Autodesk Inventor part; units mm, degrees
ref_plane "YZ Plane" through (0, 0, 0) normal (1, 0, 0) x (0, 1, 0)
ref_plane "XZ Plane" through (0, 0, 0) normal (0, 1, 0) x (-1, 0, 0)
ref_plane "XY Plane" through (0, 0, 0) normal (0, 0, 1) x (1, 0, 0)
sketch "スケッチ1" plane through (0, 0, 0) normal (0, 0, 1) x (1, 0, 0)
  arc A0 (-3.8168, 9.7817) -> (-3.6234, 7.4117) centre (4.2362, 9.2462) ccw
  arc A1 (-3.6234, 7.4117) -> (-4.2231, 7.0872) centre (0, 0) ccw
  arc A2 (-4.2231, 7.0872) -> (-6.1013, 8.5454) centre (-10.0576, 1.5108) ccw
  arc A3 (-6.1013, 8.5454) -> (-6.7861, 8.0124) centre (0, 0) ccw
  arc A4 (-6.7861, 8.0124) -> (-5.8336, 5.8336) centre (1.0044, 10.1207) ccw
  arc A5 (-5.8336, 5.8336) -> (-6.2954, 5.332) centre (0, 0) ccw
  arc A6 (-6.2954, 5.332) -> (-8.5454, 6.1013) centre (-10.0032, -1.8368) ccw
  arc A7 (-8.5454, 6.1013) -> (-9.0201, 5.3748) centre (0, 0) ccw
  arc A8 (-9.0201, 5.3748) -> (-7.4117, 3.6234) centre (-2.3362, 9.8985) ccw
  arc A9 (-7.4117, 3.6234) -> (-7.6856, 2.9989) centre (0, 0) ccw
  arc A10 (-7.6856, 2.9989) -> (-10.0635, 2.996) centre (-8.8648, -4.9853) ccw
  arc A11 (-10.0635, 2.996) -> (-10.2765, 2.1548) centre (0, 0) ccw
  arc A12 (-10.2765, 2.1548) -> (-8.1866, 1.0205) centre (-5.4236, 8.6036) ccw
  arc A13 (-8.1866, 1.0205) -> (-8.243, 0.3409) centre (0, 0) ccw
  arc A14 (-8.243, 0.3409) -> (-10.491, -0.4339) centre (-6.7658, -7.5935) ccw
  arc A15 (-10.491, -0.4339) -> (-10.4194, -1.2988) centre (0, 0) ccw
  arc A16 (-10.4194, -1.2988) -> (-8.0744, -1.693) centre (-7.9233, 6.3764) ccw
  arc A17 (-8.0744, -1.693) -> (-7.907, -2.354) centre (0, 0) ccw
  arc A18 (-7.907, -2.354) -> (-9.7817, -3.8168) centre (-3.9336, -9.3789) ccw
  arc A19 (-9.7817, -3.8168) -> (-9.4331, -4.6116) centre (0, 0) ccw
  arc A20 (-9.4331, -4.6116) -> (-7.0872, -4.2231) centre (-9.5644, 3.4582) ccw
  arc A21 (-7.0872, -4.2231) -> (-6.7143, -4.7939) centre (0, 0) ccw
  arc A22 (-6.7143, -4.7939) -> (-8.0124, -6.7861) centre (-0.6751, -10.148) ccw
  arc A23 (-8.0124, -6.7861) -> (-7.4246, -7.4246) centre (0, 0) ccw
  arc A24 (-7.4246, -7.4246) -> (-5.332, -6.2954) centre (-10.1691, 0.1652) ccw
  arc A25 (-5.332, -6.2954) -> (-4.7939, -6.7143) centre (0, 0) ccw
  arc A26 (-4.7939, -6.7143) -> (-5.3748, -9.0201) centre (2.6565, -9.8173) ccw
  arc A27 (-5.3748, -9.0201) -> (-4.6116, -9.4331) centre (0, 0) ccw
  arc A28 (-4.6116, -9.4331) -> (-2.9989, -7.6856) centre (-9.6717, -3.1456) ccw
  arc A29 (-2.9989, -7.6856) -> (-2.354, -7.907) centre (0, 0) ccw
  arc A30 (-2.354, -7.907) -> (-2.1548, -10.2765) centre (5.7003, -8.4228) ccw
  arc A31 (-2.1548, -10.2765) -> (-1.2988, -10.4194) centre (0, 0) ccw
  arc A32 (-1.2988, -10.4194) -> (-0.3409, -8.243) centre (-8.1263, -6.1156) ccw
  arc A33 (-0.3409, -8.243) -> (0.3409, -8.243) centre (0, 0) ccw
  arc A34 (0.3409, -8.243) -> (1.2988, -10.4194) centre (8.1263, -6.1156) ccw
  arc A35 (1.2988, -10.4194) -> (2.1548, -10.2765) centre (0, 0) ccw
  arc A36 (2.1548, -10.2765) -> (2.354, -7.907) centre (-5.7003, -8.4228) ccw
  arc A37 (2.354, -7.907) -> (2.9989, -7.6856) centre (0, 0) ccw
  arc A38 (2.9989, -7.6856) -> (4.6116, -9.4331) centre (9.6717, -3.1456) ccw
  arc A39 (4.6116, -9.4331) -> (5.3748, -9.0201) centre (0, 0) ccw
  arc A40 (5.3748, -9.0201) -> (4.7939, -6.7143) centre (-2.6565, -9.8173) ccw
  arc A41 (4.7939, -6.7143) -> (5.332, -6.2954) centre (0, 0) ccw
  arc A42 (5.332, -6.2954) -> (7.4246, -7.4246) centre (10.1691, 0.1652) ccw
  arc A43 (7.4246, -7.4246) -> (8.0124, -6.7861) centre (0, 0) ccw
  arc A44 (8.0124, -6.7861) -> (6.7143, -4.7939) centre (0.6751, -10.148) ccw
  arc A45 (6.7143, -4.7939) -> (7.0872, -4.2231) centre (0, 0) ccw
  arc A46 (7.0872, -4.2231) -> (9.4331, -4.6116) centre (9.5644, 3.4582) ccw
  arc A47 (9.4331, -4.6116) -> (9.7817, -3.8168) centre (0, 0) ccw
  arc A48 (9.7817, -3.8168) -> (7.907, -2.354) centre (3.9336, -9.3789) ccw
  arc A49 (7.907, -2.354) -> (8.0744, -1.693) centre (0, 0) ccw
  arc A50 (8.0744, -1.693) -> (10.4194, -1.2988) centre (7.9233, 6.3764) ccw
  arc A51 (10.4194, -1.2988) -> (10.491, -0.4339) centre (0, 0) ccw
  arc A52 (10.491, -0.4339) -> (8.243, 0.3409) centre (6.7658, -7.5935) ccw
  arc A53 (8.243, 0.3409) -> (8.1866, 1.0205) centre (0, 0) ccw
  arc A54 (8.1866, 1.0205) -> (10.2765, 2.1548) centre (5.4236, 8.6036) ccw
  arc A55 (10.2765, 2.1548) -> (10.0635, 2.996) centre (0, 0) ccw
  arc A56 (10.0635, 2.996) -> (7.6856, 2.9989) centre (8.8648, -4.9853) ccw
  arc A57 (7.6856, 2.9989) -> (7.4117, 3.6234) centre (0, 0) ccw
  arc A58 (7.4117, 3.6234) -> (9.0201, 5.3748) centre (2.3362, 9.8985) ccw
  arc A59 (9.0201, 5.3748) -> (8.5454, 6.1013) centre (0, 0) ccw
  arc A60 (8.5454, 6.1013) -> (6.2954, 5.332) centre (10.0032, -1.8368) ccw
  arc A61 (6.2954, 5.332) -> (5.8336, 5.8336) centre (0, 0) ccw
  arc A62 (5.8336, 5.8336) -> (6.7861, 8.0124) centre (-1.0044, 10.1207) ccw
  arc A63 (6.7861, 8.0124) -> (6.1013, 8.5454) centre (0, 0) ccw
  arc A64 (6.1013, 8.5454) -> (4.2231, 7.0872) centre (10.0576, 1.5108) ccw
  arc A65 (4.2231, 7.0872) -> (3.6234, 7.4117) centre (0, 0) ccw
  arc A66 (3.6234, 7.4117) -> (3.8168, 9.7817) centre (-4.2362, 9.2462) ccw
  arc A67 (3.8168, 9.7817) -> (2.996, 10.0635) centre (0, 0) ccw
  arc A68 (2.996, 10.0635) -> (1.693, 8.0744) centre (9.0221, 4.6946) ccw
  arc A69 (1.693, 8.0744) -> (1.0205, 8.1866) centre (0, 0) ccw
  arc A70 (1.0205, 8.1866) -> (0.4339, 10.491) centre (-7.0089, 7.3697) ccw
  arc A71 (0.4339, 10.491) -> (-0.4339, 10.491) centre (0, 0) ccw
  arc A72 (-0.4339, 10.491) -> (-1.0205, 8.1866) centre (7.0089, 7.3697) ccw
  arc A73 (-1.0205, 8.1866) -> (-1.693, 8.0744) centre (0, 0) ccw
  arc A74 (-1.693, 8.0744) -> (-2.996, 10.0635) centre (-9.0221, 4.6946) ccw
  arc A75 (-2.996, 10.0635) -> (-3.8168, 9.7817) centre (0, 0) ccw
  line L0 (-2, 1.5) -> (2, 1.5)
  line L1 (2, -1.5) -> (-2, -1.5)
  arc A76 (2, -1.5) -> (2, 1.5) centre (0, 0) ccw
  arc A77 (-2, 1.5) -> (-2, -1.5) centre (0, 0) ccw
  point P0 (0, 0)
  point P1 (0, 0)
  point P2 (0, 0)
  point P3 (0, 0)
  point P4 (0, 0)
  point P5 (0, 0)
  point P6 (0, 0)
  point P7 (0, 0)
  point P8 (0, 0)
  point P9 (0, 0)
  point P10 (0, 0)
  point P11 (0, 0)
  point P12 (0, 0)
  point P13 (0, 0)
  point P14 (0, 0)
  point P15 (0, 0)
  point P16 (0, 0)
  point P17 (0, 0)
  point P18 (0, 0)
  point P19 (0, 0)
  point P20 (0, 0)
  point P21 (0, 0)
  point P22 (0, 0)
  point P23 (0, 0)
  point P24 (0, 0)
  point P25 (0, 0)
  point P26 (0, 0)
  point P27 (0, 0)
  point P28 (0, 0)
  point P29 (0, 0)
  point P30 (0, 0)
  point P31 (0, 0)
  point P32 (0, 0)
  point P33 (0, 0)
  point P34 (0, 0)
extrude "押し出し1" add sketch "スケッチ1" along normal blind 6.5
properties part number "Gear19"
Design review of the part built by this model. Coordinates are the model's own, in mm. A direction names the side the tool comes from. Coordinates: 2 decimals unless noted, no trailing zeros. Order: outer loops, then holes, each group sorted by start corner. A loop starts at its lowest first (then second) coordinate and runs counter-clockwise, first axis right, second up.
Item 1: For line 1 (X direction, y = 9.5, z = 3.5); line 2 (X direction, y = 9, z = 6.25); line 3 (X direction, y = -9.5, z = 4.5), list the stretches that pass through material, from the lowest coordinate up.
Item 2: For faces 1 (the cylindrical face through (-5.174, -7.862, 3.204)), 2 (the cylindrical face through (-2.28, 9.13, 3.2)), 3 (the cylindrical face through (-9.259, 1.502, 3.204)), 4 (the cylindrical face through (8.89, -3.01, 3.2)), list the 3-axis set-ups (+Z, -Z, +X, -X, +Y, -Y) from which the entire face can be reached by the end or side of a thin tool; tool diameter is ignored.
Item 3: Take a section at B-B, the plane y = -8.5. Write out the cut boundary in (x, z).
Item 4: Take a section at A-A, the plane y = -1. Write out the cut boundary in (x, z), then the cut area to 3 significant figures.
Item 5: The part is to be moulded in two halves that separate along Y. For faces 5 (the cylindrical face through (-9.41, 0.03, 3.2)), 6 (the cylindrical face through (-0.73, -9.35, 3.2)), 7 (the cylindrical face through (-10.18, 2.57, 3.2)), say which applies: pulls with the +Y half, pulls with the -Y half, needs draft (parallel to the pull), parting line crosses it, or undercut.
Item 6: For pin 1 Ø1 at (x, y) = (1, 6.5) entering from -Z; pin 2 Ø1.5 at (y, z) = (3, 2.5) entering from -X, all flat-tipped, find the tip position at first contact; note any pin that passes through.
Item 7: Take a section at C-C, the plane y = 6.75. Write out the cut boundary in (x, z).
The answers:
1. line 1: x = -3.83 to -2.54, -0.78 to 0.78, 2.54 to 3.83
1. line 2: x = -3.83 to -2.2, -0.9 to 0.9, 2.2 to 3.83
1. line 3: x = -2.3 to -0.8, 0.8 to 2.3
2. face 1: +Z, -Z
2. face 2: +Z, -Z, +Y
2. face 3: +Z, -Z, -X
2. face 4: +Z, -Z, +X
3. outline: (-5.31, 0) - (-3.63, 0) - (-3.63, 6.5) - (-5.31, 6.5) - close; (-2.37, 0) - (-0.42, 0) - (-0.42, 6.5) - (-2.37, 6.5) - close; (0.42, 0) - (2.37, 0) - (2.37, 6.5) - (0.42, 6.5) - close; (3.63, 0) - (5.31, 0) - (5.31, 6.5) - (3.63, 6.5) - close
4. outline: (-10.45, 0) - (-2.29, 0) - (-2.29, 6.5) - (-10.45, 6.5) - close; (2.29, 0) - (10.45, 0) - (10.45, 6.5) - (2.29, 6.5) - close
4. area: 106 mm2
5. face 5: undercut
5. face 6: pulls with the -Y half
5. face 7: pulls with the +Y half
6. pin 1: stops at z = 0
6. pin 2: stops at x = -10.26
7. outline: (-6.33, 0) - (6.33, 0) - (6.33, 6.5) - (-6.33, 6.5) - close
